```python
from build123d import *

# Parameters (mm, degrees)
SKETCH1_W           = 50
SKETCH1_H           = 110
SKETCH1_R           = 7
SKETCH1_R_2         = 1.5
BOSS_EXTRUDE1_DEPTH = 3.175
CUT_EXTRUDE1_DEPTH  = 10


with BuildPart() as part:
    # Sketch1 → Boss-Extrude1 (new body)
    with BuildSketch(Plane(origin=(0, 0, 0), x_dir=(1, 0, 0), z_dir=(0, 1, 0))):
        with Locations((25, 55)):
            Rectangle(SKETCH1_W, SKETCH1_H)
        with Locations(Location((35, 55, 0), (0, 0, 270))):
            Circle(SKETCH1_R, mode=Mode.SUBTRACT)
        with Locations(Location((41.423632142, 62.307271214, 0), (0, 0, 270))):
            Circle(SKETCH1_R_2, mode=Mode.SUBTRACT)
        with Locations(Location((41.423331921, 46.807271217, 0), (0, 0, 270))):
            Circle(SKETCH1_R_2, mode=Mode.SUBTRACT)
        with Locations(Location((27.999788054, 39.057531217, 0), (0, 0, 270))):
            Circle(SKETCH1_R_2, mode=Mode.SUBTRACT)
        with Locations(Location((14.576544409, 46.807791215, 0), (0, 0, 270))):
            Circle(SKETCH1_R_2, mode=Mode.SUBTRACT)
        with Locations(Location((14.57684463, 62.307791212, 0), (0, 0, 270))):
            Circle(SKETCH1_R_2, mode=Mode.SUBTRACT)
        with Locations(Location((28.000388497, 70.057531211, 0), (0, 0, 270))):
            Circle(SKETCH1_R_2, mode=Mode.SUBTRACT)
    extrude(amount=BOSS_EXTRUDE1_DEPTH)

    # Sketch2 → Cut-Extrude1 (cut)
    with BuildSketch(Plane(origin=(0, 3.175, 0), x_dir=(1, 0, 0), z_dir=(0, 1, 0))):
        with BuildLine():
            Line((10, 3.25), (20, 3.25))
            ThreePointArc((20, 3.25), (22.25, 5.5), (20, 7.75))
            Line((20, 7.75), (10, 7.75))
            ThreePointArc((10, 7.75), (7.75, 5.5), (10, 3.25))
        make_face()
        with BuildLine():
            Line((10, 36.25), (20, 36.25))
            ThreePointArc((20, 36.25), (22.25, 38.5), (20, 40.75))
            Line((20, 40.75), (10, 40.75))
            ThreePointArc((10, 40.75), (7.75, 38.5), (10, 36.25))
        make_face()
        with BuildLine():
            Line((10, 69.25), (20, 69.25))
            ThreePointArc((20, 69.25), (22.25, 71.5), (20, 73.75))
            Line((20, 73.75), (10, 73.75))
            ThreePointArc((10, 73.75), (7.75, 71.5), (10, 69.25))
        make_face()
        with BuildLine():
            Line((10, 102.25), (20, 102.25))
            ThreePointArc((20, 102.25), (22.25, 104.5), (20, 106.75))
            Line((20, 106.75), (10, 106.75))
            ThreePointArc((10, 106.75), (7.75, 104.5), (10, 102.25))
        make_face()
    extrude(amount=-CUT_EXTRUDE1_DEPTH, mode=Mode.SUBTRACT)


solid = part.part
```
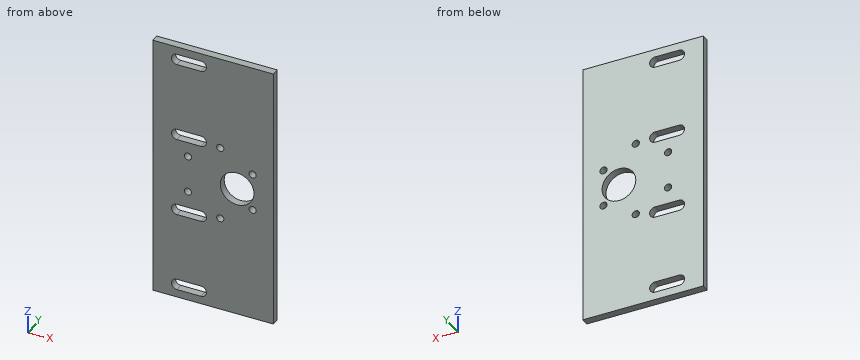
Design review of the part built by this model. Coordinates are the model's own, in mm. Round coordinates to 2 decimals unless told otherwise and drop trailing zeros. Write each loop counter-clockwise with the first axis right and the second up, starting at its lowest first coordinate (ties: lowest second). Pieces come first, ordered by that corner, then holes.
Item 1: For probe 1 along Z at (x, y) = (18.5, 0.6); probe 2 along Z at (x, y) = (8.5, 1.95); probe 3 along X at (y, z) = (1.35, -5.5), list the stretches that pass through material, from the lowest coordinate up.
Item 2: We need section A-A on z = -104.5. Write out the cut boundary in (x, y) (3 decimals), and give its area (3 significant figures).
Item 3: We need section D-D on z = -55. Write out the cut boundary in (x, y) (3 decimals), and give its area (3 significant figures).
Item 4: We need section C-C on y = 1.85. State how many separate pieces and enclosed holes the cut face has, and give its area (3 significant figures).
Item 5: We need section B-B on x = 17.5. Write out the cut boundary in (y, z) (3 decimals).
Item 6: Clearance check with a flat-ended pin moving along its axis: pin 1 Ø5 at (x, z) = (14.58, -62.31) entering from +Y (3 decimals). State where the tip first meets the part, or that it passes through.
Returned:
1. probe 1: z = -110 to -106.75, -102.25 to -73.75, -69.25 to -40.75, -36.25 to -7.75, -3.25 to 0
1. probe 2: z = -110 to -106.18, -102.82 to -73.18, -69.82 to -40.18, -36.82 to -7.18, -3.82 to 0
1. probe 3: x = 0 to 7.75, 22.25 to 50
2. outline: (0, 0) - (7.75, 0) - (7.75, 3.175) - (0, 3.175) - close; (22.25, 0) - (50, 0) - (50, 3.175) - (22.25, 3.175) - close
2. area: 113 mm2
3. outline: (0, 0) - (28, 0) - (28, 3.175) - (0, 3.175) - close; (42, 0) - (50, 0) - (50, 3.175) - (42, 3.175) - close
3. area: 114 mm2
4. separate pieces: 1
4. enclosed holes: 11
4. area: 5,060 mm2
5. outline: (0, -110) - (3.175, -110) - (3.175, -106.75) - (0, -106.75) - close; (0, -102.25) - (3.175, -102.25) - (3.175, -73.75) - (0, -73.75) - close; (0, -69.25) - (3.175, -69.25) - (3.175, -40.75) - (0, -40.75) - close; (0, -36.25) - (3.175, -36.25) - (3.175, -7.75) - (0, -7.75) - close; (0, -3.25) - (3.175, -3.25) - (3.175, 0) - (0, 0) - close
6. pin 1: stops at y = 3.175
